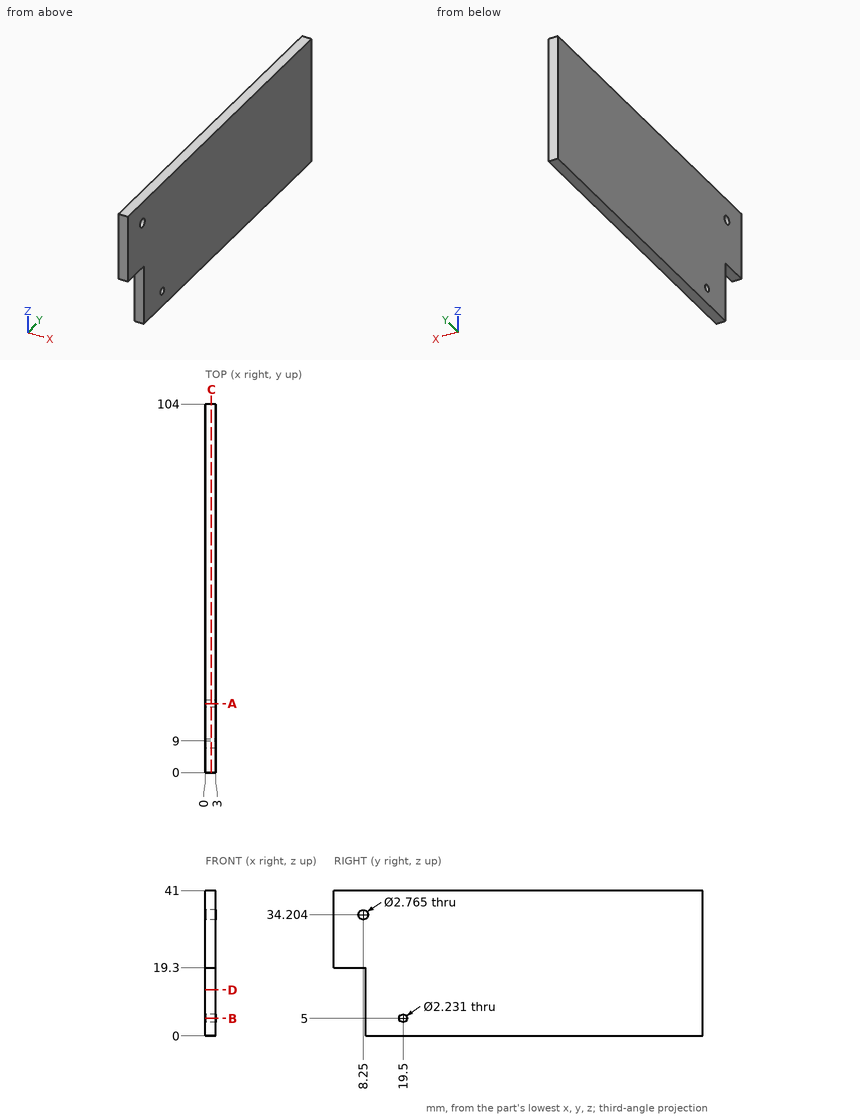
Geometry: see drawing. Coordinates: mm, zero at the bounding-box minimum. Give positions to 0.01 mm unless a question says otherwise; leave off trailing zeros. Write each loop counter-clockwise with the first axis right and the second up, starting at its lowest first coordinate (ties: lowest second). Pieces come first, ordered by that corner, then holes. Notation, with made-up numbers: (14, 89.5) - (20, 89.5) arc R19 ccw to (20, 118.5) - close; hole circle Ø9 at (81.25, 25). An arc over 180 degrees is marked (long way). Return JSON: item names as keys, results as strings. Group by question number.
1) Section C-C on x = 1.7. State how many separate pieces and enclosed holes the cut face has, plus the area to 3 significant figures.
2) Section A-A on y = 19.5. Return the cut outline in (x, z) (1 decimal), plus the area to 3 significant figures.
3) Line query: line 1 (Y direction, x = 1.8, z = 5) (1 decimal); line 2 (Z direction, x = 0.6, y = 19.5) (1 decimal); line 3 (Z direction, x = 2.1, y = 8.25). Output: solid intervals per line, ascending.
4) Section D-D on z = 13. Return the cut outline in (x, y), plus the area to 3 significant figures.
5) Section B-B on z = 5. Return the cut outline in (x, y) (1 decimal).
6) First-contact query: P1, Ø3, axis at y = 30, z = 7, coming from the -X side; P2, Ø0.9, axis at x = 2, z = 10, coming from the -Y side. Flat tips, straight axial feed; report the tip coordinate or a pass-through.
Filled in:
{
 "1": {"separate pieces": "1", "enclosed holes": "2", "area": "4,080 mm^2"},
 "2": {"outline": "(0, 0) - (3, 0) - (3, 3.9) - (0, 3.9) - close; (0, 6.1) - (3, 6.1) - (3, 41) - (0, 41) - close", "area": "116 mm^2"},
 "3": {"line 1": "y = 9 to 18.4, 20.6 to 104", "line 2": "z = 0 to 3.9, 6.1 to 41", "line 3": "z = 19.3 to 32.82, 35.59 to 41"},
 "4": {"outline": "(0, 9) - (3, 9) - (3, 104) - (0, 104) - close", "area": "285 mm^2"},
 "5": {"outline": "(0, 9) - (3, 9) - (3, 18.4) - (0, 18.4) - close; (0, 20.6) - (3, 20.6) - (3, 104) - (0, 104) - close"},
 "6": {"P1": "stops at x = 0", "P2": "stops at y = 9"}
}
